Could you check a few things on this model? Use its own coordinates, in mm. Face numbers are marked on the shaded views. A direction names the side the tool comes from. Coordinates: 2 decimals unless noted, no trailing zeros. Loops run counter-clockwise (first coordinate to the right, second up) from the corner with the lowest first, then second, coordinate; pieces in that order, holes last.
1) Imagine slicing it at A-A on x = 0. Please give me the cut outline in (y, z).
2) Thinking about a two-plate mould opening in X: for the marked faces 1, 2 and 3, which applies, released by +X, released by -X, zero draft, split by the parting line, or undercut?
3) Imagine slicing it at B-B on y = 3. Please give me the cut outline in (x, z).
4) Will these pins go through, and if not, where does the flat tip stop? P1, Ø8, axis at x = 13.86, z = 10.79, coming from the -Y side; P2, Ø4.5, axis at x = 0, z = 0, coming from the -Y side.
5) For the marked faces 4 and 5, which set-ups out of +Z, -Z, +X, -X, +Y, -Y let a thin tool reach every point of the face, with its end or its side?
6) Imagine slicing it at C-C on z = 12.7. Please give me the cut outline in (x, y).
7) If I drill on line 1 along X through (y, z) = (1.25, 8); line 2 along X through (y, z) = (5.5, 13.5); line 3 along X through (y, z) = (5.5, 8.5), over which ranges is the centre line in solid material (lowest first)?
8) Imagine slicing it at D-D on x = 12. Please give me the cut outline in (y, z).
```python
from build123d import *

# Parameters (mm, degrees)
SKETCH1_W               = 50.8
SKETCH1_H               = 50.8
BOSS_EXTRUDE1_DEPTH     = 6.35
F_8_CLEARANCE_HOLE1_D   = 4.4958
F_1_4_CLEARANCE_HOLE1_D = 6.7564
CUT_EXTRUDE1_DEPTH      = 4.064
SKETCH9_R               = 2.38125
CUT_EXTRUDE2_DEPTH      = 37.477972806


with BuildPart() as part:
    # Sketch1 → Boss-Extrude1 (new body)
    with BuildSketch(Plane(origin=(0, 0, 0), x_dir=(1, 0, 0), z_dir=(0, 1, 0))):
        Rectangle(SKETCH1_W, SKETCH1_H)
    extrude(amount=BOSS_EXTRUDE1_DEPTH)

    # #8 Clearance Hole1 (through all)
    with Locations(Plane(origin=(0, 6.35, 0), x_dir=(1, 0, 0), z_dir=(0, 1, 0))):
        with Locations((-18.288, 12.7), (18.288, 12.7), (0, -12.7)):
            Hole(F_8_CLEARANCE_HOLE1_D / 2)

    # 1/4 Clearance Hole1 (through all)
    with Locations(Plane(origin=(0, 6.35, 0), x_dir=(1, 0, 0), z_dir=(0, 1, 0))):
        with Locations((0, 14.61008), (-13.86078, -10.78992), (13.86078, -10.78992)):
            Hole(F_1_4_CLEARANCE_HOLE1_D / 2)

    # Sketch8 → Cut-Extrude1 (cut)
    with BuildSketch(Plane.XZ):
        with BuildLine():
            Line((-19.44878, 16.37792), (-19.44878, 5.20192))
            ThreePointArc((-19.44878, 5.20192), (-13.86078, -0.38608), (-8.27278, 5.20192))
            Line((-8.27278, 5.20192), (-8.27278, 16.37792))
            ThreePointArc((-8.27278, 16.37792), (-13.86078, 21.96592), (-19.44878, 16.37792))
        make_face()
        with BuildLine():
            Line((8.27278, 16.37792), (8.27278, 5.20192))
            ThreePointArc((8.27278, 5.20192), (13.86078, -0.38608), (19.44878, 5.20192))
            Line((19.44878, 5.20192), (19.44878, 16.37792))
            ThreePointArc((19.44878, 16.37792), (13.86078, 21.96592), (8.27278, 16.37792))
        make_face()
        with BuildLine():
            Line((-5.588, -9.02208), (5.588, -9.02208))
            ThreePointArc((5.588, -9.02208), (11.176, -14.61008), (5.588, -20.19808))
            Line((5.588, -20.19808), (-5.588, -20.19808))
            ThreePointArc((-5.588, -20.19808), (-11.176, -14.61008), (-5.588, -9.02208))
        make_face()
    extrude(amount=-CUT_EXTRUDE1_DEPTH, mode=Mode.SUBTRACT)

    # Sketch9 → Cut-Extrude2 (cut, through all)
    with BuildSketch(Plane(origin=(0, 6.35, 0), x_dir=(1, 0, 0), z_dir=(0, 1, 0))):
        with Locations(Location((0, 0, 0), (0, 0, 270))):
            Circle(SKETCH9_R)
    extrude(amount=-CUT_EXTRUDE2_DEPTH, mode=Mode.SUBTRACT)


solid = part.part
```
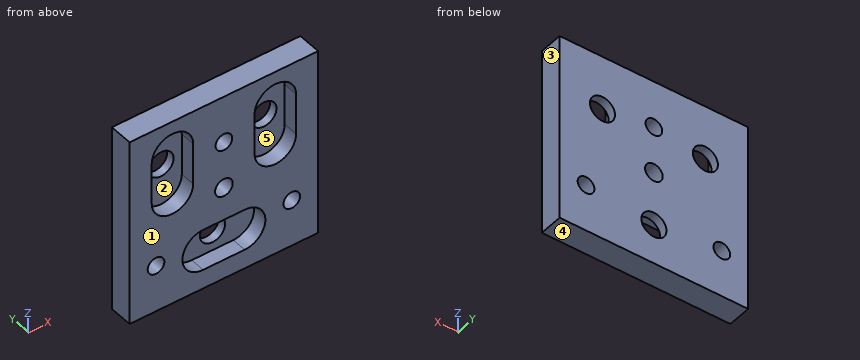
Filled in:
1. outline: (0, -25.4) - (6.35, -25.4) - (6.35, -17.99) - (4.06, -17.99) - (4.06, -20.2) - (0, -20.2) - close; (0, -9.02) - (4.06, -9.02) - (4.06, -11.23) - (6.35, -11.23) - (6.35, -2.38) - (0, -2.38) - close; (0, 2.38) - (6.35, 2.38) - (6.35, 10.45) - (0, 10.45) - close; (0, 14.95) - (6.35, 14.95) - (6.35, 25.4) - (0, 25.4) - close
2. face 1: zero draft
2. face 2: undercut
2. face 3: released by +X
3. outline: (-25.4, -25.4) - (25.4, -25.4) - (25.4, 25.4) - (-25.4, 25.4) - close; hole circle Ø4.5 at (-18.29, -12.7); hole (-19.45, 5.2) arc R5.59 ccw to (-8.27, 5.2) - (-8.27, 16.38) arc R5.59 ccw to (-19.45, 16.38) - close; hole (-5.59, -20.2) - (5.59, -20.2) arc R5.59 ccw to (5.59, -9.02) - (-5.59, -9.02) arc R5.59 ccw to start; hole circle Ø4.76 at (0, 0); hole circle Ø4.5 at (0, 12.7); hole (8.27, 5.2) arc R5.59 ccw to (19.45, 5.2) - (19.45, 16.38) arc R5.59 ccw to (8.27, 16.38) - close; hole circle Ø4.5 at (18.29, -12.7)
4. P1: stops at y = 4.06
4. P2: passes through
5. face 4: -Z, +X, -X, +Y, -Y
5. face 5: -Y
6. outline: (-25.4, 0) - (-19.45, 0) - (-19.45, 4.06) - (-16.65, 4.06) - (-16.65, 6.35) - (-25.4, 6.35) - close; (-11.07, 4.06) - (-8.27, 4.06) - (-8.27, 0) - (-2.25, 0) - (-2.25, 6.35) - (-11.07, 6.35) - close; (2.25, 0) - (8.27, 0) - (8.27, 4.06) - (11.07, 4.06) - (11.07, 6.35) - (2.25, 6.35) - close; (16.65, 4.06) - (19.45, 4.06) - (19.45, 0) - (25.4, 0) - (25.4, 6.35) - (16.65, 6.35) - close
7. line 1: x = -25.4 to -19.45, -8.27 to 8.27, 19.45 to 25.4
7. line 2: x = -25.4 to -15.88, -11.84 to -2.1, 2.1 to 11.84, 15.88 to 25.4
7. line 3: x = -25.4 to -16.34, -11.38 to 11.38, 16.34 to 25.4
8. outline: (0, -25.4) - (6.35, -25.4) - (6.35, 7.97) - (4.06, 7.97) - (4.06, -0.07) - (0, -0.07) - close; (0, 21.65) - (4.06, 21.65) - (4.06, 13.61) - (6.35, 13.61) - (6.35, 25.4) - (0, 25.4) - close
